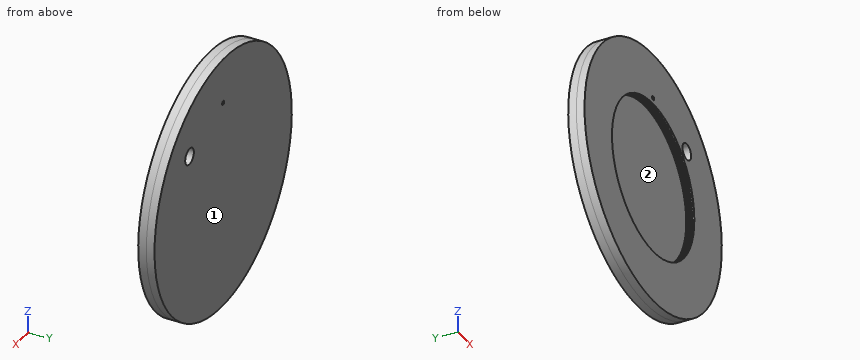
from build123d import *

# Parameters (mm, degrees)
SKETCH1_R               = 15.875
BOSS_EXTRUDE1_DEPTH     = 1
BOSS_EXTRUDE2_START     = 1
SKETCH2_R               = 15.875
SKETCH2_R_2             = 9.525
BOSS_EXTRUDE2_DEPTH     = 1
THREAD1_PITCH           = 0.25
CUT_EXTRUDE1_DEPTH      = 23.539548638
CUT_EXTRUDE1_DEPTH_BACK = 23.539548638
SKETCH3_R               = 0.25
CUT_EXTRUDE2_DEPTH      = 23.539548576
CUT_EXTRUDE2_DEPTH_BACK = 23.539548576
SKETCH4_R               = 1


with BuildPart() as part:
    # Sketch1 → Boss-Extrude1 (new body)
    with BuildSketch(Plane(origin=(0, 0, 0), x_dir=(1, 0, 0), z_dir=(0, 1, 0))):
        with Locations(Location((0, 0, 0), (0, 0, 270))):
            Circle(SKETCH1_R)
    extrude(amount=BOSS_EXTRUDE1_DEPTH)

    # Sketch2 → Boss-Extrude2 (add)
    with BuildSketch(Plane.XZ.offset(BOSS_EXTRUDE2_START)):
        with Locations(Location((0, 0, 0), (0, 0, 270))):
            Circle(SKETCH2_R)
        with Locations(Location((0, 0, 0), (0, 0, 270))):
            Circle(SKETCH2_R_2, mode=Mode.SUBTRACT)
    extrude(amount=-BOSS_EXTRUDE2_DEPTH)

    # Thread1: the profile of Thread Profile1 profile screwed along a right-hand helix of 4 turns, 6 arcs to a turn; built about Z, then put on its axis
    thread1_z = Axis((0, 0, 0), (0, 0, 1))
    thread1_corners = [(9.5247, 0, -0.000173205), (9.660316469, 0, 0.078125), (9.660316469, 0, 0.109375), (9.5247, 0, 0.187673204)]
    with BuildLine(mode=Mode.PRIVATE) as thread1_profile:
        Line(thread1_corners[0], thread1_corners[1])
        Line(thread1_corners[1], thread1_corners[2])
        Line(thread1_corners[2], thread1_corners[3])
        Line(thread1_corners[3], thread1_corners[0])
    thread1_cap = Face(thread1_profile.wire())
    thread1_turn_angles = [0, 30, 60, 90, 120, 150, 180, 210, 240, 270, 300, 330, 360]
    thread1_turn_weights = [1, 0.8660254037844387, 1, 0.8660254037844387, 1, 0.8660254037844387, 1, 0.8660254037844387, 1, 0.8660254037844387, 1, 0.8660254037844387, 1]
    thread1_turn_rails = [Edge.make_bspline([Vector(p[0], p[1], 0).rotate(thread1_z, thread1_turn_angles[k]) / thread1_turn_weights[k] + Vector(0, 0, p[2] + THREAD1_PITCH * thread1_turn_angles[k] / 360) for k in range(13)], [0, 0, 0, 1, 1, 2, 2, 3, 3, 4, 4, 5, 5, 6, 6, 6], 2, thread1_turn_weights) for p in thread1_corners]
    thread1_turn_sides = [Face.make_surface_from_curves(thread1_turn_rails[p[0]], thread1_turn_rails[p[1]]) for p in [(0, 1), (1, 2), (2, 3), (3, 0)]]
    thread1 = Plane(origin=(0, -1, 0), x_dir=(1, 0, 0), z_dir=(0, 1, 0)) * Solid(Shell([*[p.moved(Location((0, 0, THREAD1_PITCH * i))) for i in range(4) for p in thread1_turn_sides], thread1_cap, thread1_cap.rotate(thread1_z, 1440).moved(Location((0, 0, THREAD1_PITCH * 1440 / 360)))]))
    add(thread1, mode=Mode.SUBTRACT)

    # Sketch3 → Cut-Extrude1 (cut, two sides: drawn at the far end of the back side and taken through both)
    with BuildSketch(Plane(origin=(0, 1, 0), x_dir=(1, 0, 0), z_dir=(0, 1, 0)).offset(-CUT_EXTRUDE1_DEPTH_BACK)):
        with Locations(Location((0, -10.25, 0), (0, 0, 270))):
            Circle(SKETCH3_R)
    extrude(amount=CUT_EXTRUDE1_DEPTH + CUT_EXTRUDE1_DEPTH_BACK, mode=Mode.SUBTRACT)

    # Sketch4 → Cut-Extrude2 (cut, two sides: drawn at the far end of the back side and taken through both)
    with BuildSketch(Plane.XZ.offset(1).offset(-CUT_EXTRUDE2_DEPTH_BACK)):
        with Locations(Location((7.778174593, 7.778174593, 0), (0, 0, 270))):
            Circle(SKETCH4_R)
    extrude(amount=CUT_EXTRUDE2_DEPTH + CUT_EXTRUDE2_DEPTH_BACK, mode=Mode.SUBTRACT)


solid = part.part
Source: CAD feature listing. Evaluate the final solid. Frame: model axes, mm. Face numbers are marked on the shaded views. Round coordinates to 2 decimals unless told otherwise and drop trailing zeros. Loops run counter-clockwise (first coordinate to the right, second up) from the corner with the lowest first, then second, coordinate; pieces in that order, holes last.
Q1. Section B-B, the plane z = 14.5. Return loops of the section in (x, y).
Q2. Mould query, pull axis Z, two halves, no side actions, for the marked faces 1 and 2. Classes: pulls with the +Z half, pulls with the -Z half, needs draft (parallel to the pull), parting line crosses it, or undercut.
Q3. Ray query, line 1 (Z direction, x = 0, y = -0.9) (3 decimals); line 2 (Z direction, x = 0, y = 0.45) (3 decimals); line 3 (Z direction, x = 0, y = -0.4) (3 decimals). Return the intervals inside material, ascending.
Q4. First-contact query: P1, Ø5.5, axis at x = -2.5, z = -2.5, coming from the -Y side. Flat tip, straight axial feed; report the tip coordinate or a pass-through.
Q5. Section A-A, the plane x = -11. Return loops of the section in (y, z), plus the area to 3 significant figures.
Solutions:
1. outline: (-6.46, -1) - (6.46, -1) - (6.46, 1) - (-6.46, 1) - close
2. face 1: needs draft
2. face 2: undercut
3. line 1: z = -15.875 to -9.59, 9.525 to 10, 10.5 to 15.875
3. line 2: z = -15.875 to 10, 10.5 to 15.875
3. line 3: z = -15.875 to -9.59, 9.568 to 10, 10.5 to 15.875
4. P1: stops at y = 0
5. outline: (-1, -11.45) - (1, -11.45) - (1, 11.45) - (-1, 11.45) - close
5. area: 45.8 mm2
